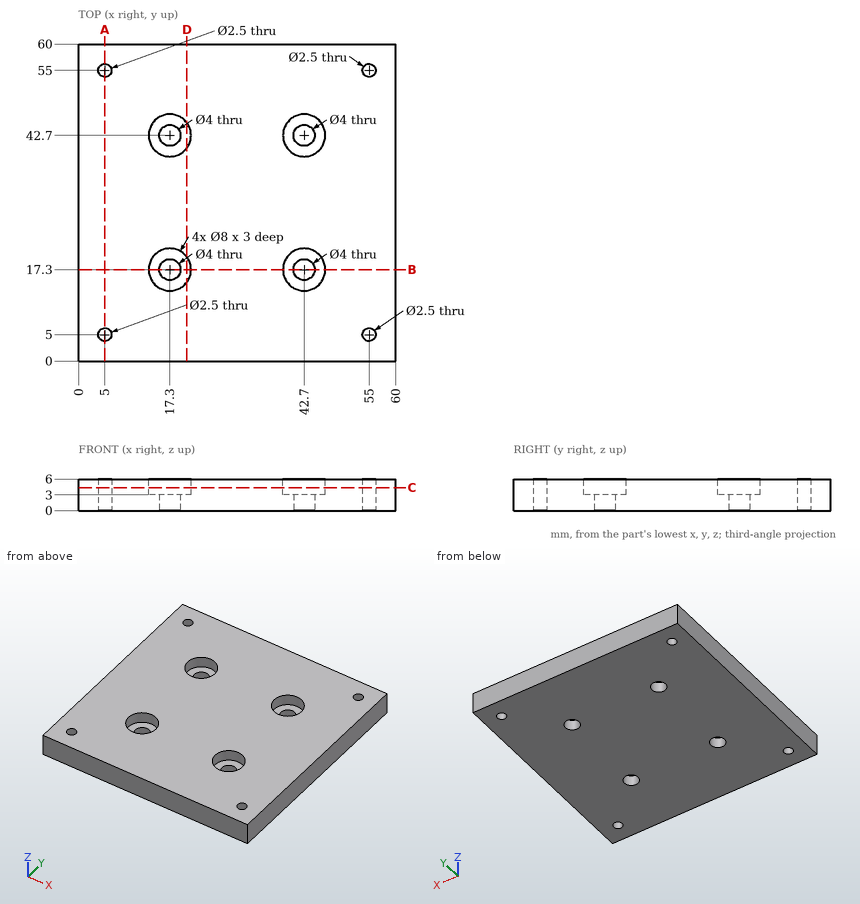
Verification items for this drawing (mm, ordinates from the low corner). Round coordinates to 2 decimals unless told otherwise and drop trailing zeros. Loops run counter-clockwise (first coordinate to the right, second up) from the corner with the lowest first, then second, coordinate; pieces in that order, holes last. Notation, with made-up numbers: (27.25, 54.25) - (68.25, 54.25) arc R18 ccw to (68.25, 81.25) - close; hole circle Ø10 at (-20.5, 27). An arc over 180 degrees is marked (long way). Answer as CSV lines item,"result". Start each with the question number.
Item 1: Depth check by flat-ended pin: P1, Ø2.5, axis at x = 42, y = 16, coming from the +Z side. Enter the tip coordinate at first touch or a pass-through.
Item 2: Section check C-C (z = 4.35). Count the separate pieces of the cut face and the enclosed holes in it, and give its area (3 significant figures).
Item 3: Scan lines: line 1 (Y direction, x = 17.3, z = 4.4); line 2 (X direction, y = 42.7, z = 2.2); line 3 (Y direction, x = 5, z = 3.7). Record each from-to range of solid material in increasing order. Write a range as [from, to].
Item 4: Section check D-D (x = 20.5). Record the boundary of the cut face in (y, z).
Item 5: Section check B-B (y = 17.3). Record the boundary of the cut face in (x, z), and give its area (3 significant figures).
Item 6: Section check A-A (x = 5). Record the boundary of the cut face in (y, z), and give its area (3 significant figures).
Report:
1,P1,"stops at z = 3"
2,separate pieces,"1"
2,enclosed holes,"8"
2,area,"3,380 mm2"
3,line 1,"y = [0, 13.3], [21.3, 38.7], [46.7, 60]"
3,line 2,"x = [0, 15.3], [19.3, 40.7], [44.7, 60]"
3,line 3,"y = [0, 3.75], [6.25, 53.75], [56.25, 60]"
4,outline,"(0, 0) - (60, 0) - (60, 6) - (45.1, 6) - (45.1, 3) - (40.3, 3) - (40.3, 6) - (19.7, 6) - (19.7, 3) - (14.9, 3) - (14.9, 6) - (0, 6) - close"
5,outline,"(0, 0) - (15.3, 0) - (15.3, 3) - (13.3, 3) - (13.3, 6) - (0, 6) - close; (19.3, 0) - (40.7, 0) - (40.7, 3) - (38.7, 3) - (38.7, 6) - (21.3, 6) - (21.3, 3) - (19.3, 3) - close; (44.7, 0) - (60, 0) - (60, 6) - (46.7, 6) - (46.7, 3) - (44.7, 3) - close"
5,area,"288 mm2"
6,outline,"(0, 0) - (3.75, 0) - (3.75, 6) - (0, 6) - close; (6.25, 0) - (53.75, 0) - (53.75, 6) - (6.25, 6) - close; (56.25, 0) - (60, 0) - (60, 6) - (56.25, 6) - close"
6,area,"330 mm2"
